Autodesk Inventor part; units mm, degrees
ref_plane "YZ Plane" through (0, 0, 0) normal (1, 0, 0) x (0, 1, 0)
ref_plane "XZ Plane" through (0, 0, 0) normal (0, 1, 0) x (-1, 0, 0)
ref_plane "XY Plane" through (0, 0, 0) normal (0, 0, 1) x (1, 0, 0)
sketch "スケッチ1" plane through (0, 0, 0) normal (1, 0, 0) x (0, 1, 0)
  line L0 (0, 0) -> (15, 0)
  line L1 (15, 0) -> (15, -10)
  line L2 (15, -10) -> (0, -10)
  line L3 (0, -10) -> (0, 0)
  line L4 (1, -1) -> (14, -1)
  line L5 (14, -1) -> (14, -9)
  line L6 (14, -9) -> (1, -9)
  line L7 (1, -9) -> (1, -1)
  dimension "d0" = 15
  dimension "d1" = 10
  dimension "d2" = 13
  dimension "d3" = 8
  dimension "d4" = 1
  dimension "d5" = 1
extrude "押し出し1" add sketch "スケッチ1" along normal blind 106
sketch "スケッチ2" plane through (0, 15, 0) normal (0, 1, 0) x (1, 0, 0)
  line L0 (0, 9) -> (0, 1)
  line L1 (0, 5) -> (120, 5)
  line L2 (106, 10) -> (106, 0)
  point P0 (0, 0)
  point P1 (5, 5)
  point P2 (101, 5)
  point P3 (106, 0)
  dimension "d8" = 5
  dimension "d9" = 5
hole "穴1" at (5, 15, -5) at (101, 15, -5) direction (0, -1, 0) diameter 3.2 end through all
properties part number "link2_pipe2" material "アルミニウム 6061"
Verification items for the finished model (mm, model axes). A direction names the side the tool comes from. Round coordinates to 2 decimals unless told otherwise and drop trailing zeros. Loops run counter-clockwise (first coordinate to the right, second up) from the corner with the lowest first, then second, coordinate; pieces in that order, holes last. Notation, with made-up numbers: (83.5, -1.5) - (112.5, -1.5) arc R28 cw to (112.5, 37.5) - close; hole circle Ø2 at (87, -28.75). An arc over 180 degrees is marked (long way). Write item = value, one per line.
Q1. Sectioned sample at D-D on x = 23.5. Record the boundary of the cut face in (y, z).
Here are the results:
outline = (0, -10) - (15, -10) - (15, 0) - (0, 0) - close; hole (1, -9) - (14, -9) - (14, -1) - (1, -1) - close
Q2. Sectioned sample at B-B on z = -2.5. Record the boundary of the cut face in (x, y), plus the area to 3 significant figures.
Here are the results:
outline = (0, 0) - (106, 0) - (106, 1) - (0, 1) - close; (0, 14) - (106, 14) - (106, 15) - (0, 15) - close
area = 212 mm^2
Q3. Sectioned sample at C-C on y = 4. Record the boundary of the cut face in (x, z).
Here are the results:
outline = (0, -10) - (106, -10) - (106, -9) - (0, -9) - close; (0, -1) - (106, -1) - (106, 0) - (0, 0) - close
Q4. Material ranges on L1, parallel to X at y = 14.7, z = -5; L2, parallel to Z at x = 70.5, y = 8; L3, parallel to Y at x = 11.5, z = -6.25, recorded low to high.
Here are the results:
L1 = 0 to 3.4, 6.6 to 99.4, 102.6 to 106
L2 = -10 to -9, -1 to 0
L3 = 0 to 1, 14 to 15
Q5. Tool access check on faces 5 (the flat face through (52, 8, -9)), 6 (the cylindrical face through (99.414, 14.493, -5.208)). Record the directions out of +Z, -Z, +X, -X, +Y, -Y that give a thin tool (end or side, any length) a straight path to the whole face; none if there is none.
Here are the results:
face_5 = +X, -X
face_6 = +Y, -Y
Q6. Depth check by flat-ended pin: pin 1 (3 mm diameter, centred on x = 101, z = -5, fed in from -Y). Enter the tip coordinate at first touch or a pass-through.
Here are the results:
pin_1 = through
Q7. Mould release check, pull along X, two halves, no side actions. Record for faces 1 (the flat face through (52, 1, -5)), 2 (the flat face through (0, 7.4, -9.4)), 3 (the cylindrical face through (99.414, 0.493, -5.208)), 4 (the flat face through (106, 7.4, -9.4)): +X half, -X half, draft (parallel to the pull), parting line (faces both ways), or undercut.
Here are the results:
face_1 = draft
face_2 = -X half
face_3 = undercut
face_4 = +X half
Q8. Sectioned sample at A-A on x = 5. Record the boundary of the cut face in (y, z).
Here are the results:
outline = (0, -10) - (15, -10) - (15, -6.6) - (14, -6.6) - (14, -9) - (1, -9) - (1, -6.6) - (0, -6.6) - close; (0, -3.4) - (1, -3.4) - (1, -1) - (14, -1) - (14, -3.4) - (15, -3.4) - (15, 0) - (0, 0) - close
